```python
from build123d import *

# Parameters (mm, degrees)
BOSS_EXTRUDE1_DEPTH       = 53.2
SKETCH2_W                 = 95
SKETCH2_H                 = 20
BOSS_EXTRUDE2_DEPTH       = 3.5
CHAMFER1_SIZE             = 50
CHAMFER1_SIZE2            = 10
SKETCH3_W                 = 89
SKETCH3_H                 = 19
BOSS_EXTRUDE3_DEPTH       = 3.5
BOSS_EXTRUDE4_START       = -3.5
BOSS_EXTRUDE4_DEPTH       = 6
FILLET1_R                 = 5
F_2_5MM_DOWEL_HOLE1_D     = 3.2
F_2_5MM_DOWEL_HOLE1_DEPTH = 6.5
F_2_5MM_DOWEL_HOLE1_TIP   = 0.96137699


with BuildPart() as part:
    # Sketch1 → Boss-Extrude1 (new body)
    with BuildSketch(Plane.XY):
        Polygon((-60.5, 15), (-60.5, 20), (-57.5, 20), (-57.5, 0), (-152.5, 0), (-152.5, 20), (-149.5, 20), (-149.5, 15), align=None)
    extrude(amount=BOSS_EXTRUDE1_DEPTH)

    # Sketch2 → Boss-Extrude2 (add)
    with BuildSketch(Plane.XY.offset(53.2)):
        with Locations((-105, 10)):
            Rectangle(SKETCH2_W, SKETCH2_H)
    extrude(amount=BOSS_EXTRUDE2_DEPTH)

    # Chamfer1
    chamfer1_edges = [part.edges().sort_by_distance(p)[0] for p in [
        (-105, 0, 56.7),
    ]]
    chamfer1_side = [part.faces().sort_by_distance(p)[0] for p in [
        (-105, 0, 28.35),
    ]]
    chamfer(chamfer1_edges, length=CHAMFER1_SIZE, length2=CHAMFER1_SIZE2, reference=chamfer1_side[0])

    # Sketch3 → Boss-Extrude3 (add)
    with BuildSketch(Plane.XY.offset(56.7)):
        with Locations((-105, 29.5)):
            Rectangle(SKETCH3_W, SKETCH3_H)
        Polygon((-152.5, 42.463842296), (-152.5, 20), (-149.5, 20), (-149.5, 39), (-60.5, 39), (-60.5, 20), (-57.5, 20), (-57.5, 42.463842296), align=None)
    extrude(amount=-BOSS_EXTRUDE3_DEPTH)

    # Sketch3<3> → Boss-Extrude4 (add)
    with BuildSketch(Plane.XY.offset(56.7).offset(BOSS_EXTRUDE4_START)):
        Polygon((-152.5, 42.463842296), (-152.5, 20), (-149.5, 20), (-149.5, 39), (-60.5, 39), (-60.5, 20), (-57.5, 20), (-57.5, 42.463842296), align=None)
    extrude(amount=-BOSS_EXTRUDE4_DEPTH)

    # Fillet1
    fillet1_edges = [part.edges().sort_by_distance(p)[0] for p in [
        (-151, 20, 47.2),
        (-59, 20, 47.2),
    ]]
    fillet(fillet1_edges, radius=FILLET1_R)

    # Ø2.5mm Dowel Hole1
    with Locations(Plane(origin=(0, 0, 0), x_dir=(-1, 0, 0), z_dir=(0, 0, -1))):
        with Locations((70, 5.6), (140, 5.6)):
            Hole(F_2_5MM_DOWEL_HOLE1_D / 2, depth=F_2_5MM_DOWEL_HOLE1_DEPTH)
            with Locations((0, 0, -(F_2_5MM_DOWEL_HOLE1_DEPTH + F_2_5MM_DOWEL_HOLE1_TIP / 2))):  # 118° drill point
                Cone(0, F_2_5MM_DOWEL_HOLE1_D / 2, F_2_5MM_DOWEL_HOLE1_TIP, mode=Mode.SUBTRACT)


solid = part.part
```
Check sheet for the modelled part. Datum: model origin and axes. Units: mm. A direction names the side the tool comes from. Round coordinates to 2 decimals unless told otherwise and drop trailing zeros. Write each loop counter-clockwise with the first axis right and the second up, starting at its lowest first coordinate (ties: lowest second). Pieces come first, ordered by that corner, then holes. Notation, with made-up numbers: (20.25, 87.25) -> (39.25, 87.25) arc R20 cw to (39.25, 91.25) -> close; hole circle Ø10 at (10, 50). An arc over 180 degrees is marked (long way). One line per question, with ' | ' between items. Start each with the question number.
1. Sectioned sample at C-C, the plane y = 21. Record the cut outline in (x, z), then the cut area to 4 significant figures.
2. Set-up check for faces 1 (the face through (-106, 0, 3)), 2 (the face through (-151, 20, 21)), 3 (the face through (-106, 39, 50)): record each of +Z, -Z, +X, -X, +Y, -Y from which the full face is reachable in a straight line by a thin tool's end or side.
3. Sectioned sample at B-B, the plane x = -118. Record the cut outline in (y, z), then the cut area to 3 significant figures.
4. Sectioned sample at D-D, the plane z = 39. Record the cut outline in (x, y).
5. Sectioned sample at A-A, the plane z = 50. Record the cut outline in (x, y), then the cut area to 3 significant figures.
6. Release check for a two-part mould opening along X. For faces 4 (the face through (-58.98, 21.43, 45.7)), 5 (the face through (-152.5, 17, 35)), 6 (the face through (-106, 27, 53.2)) record: +X half, -X half, draft (parallel to the pull), parting line (faces both ways), or undercut.
7. Depth check by flat-ended pin: pin 1 (5 mm diameter, centred on x = -86.5, z = 50, fed in from -Y); pin 2 (19 mm diameter, centred on x = -100.5, y = 37.5, fed in from -Z); pin 3 (4 mm diameter, centred on x = -97, z = 25.5, fed in from +Y). Enter the tip coordinate at first touch or a pass-through.
8. Scan lines: line 1 along X through (y, z) = (5.6, 2.75); line 2 along Y through (x, z) = (-70, 3); line 3 along X through (y, z) = (37, 49). Record each from-to range of solid material in increasing order. Write a range as from..to.
Taken from the geometry:
1) outline: (-152.5, 45.2) -> (-149.5, 45.2) -> (-149.5, 53.2) -> (-60.5, 53.2) -> (-60.5, 45.2) -> (-57.5, 45.2) -> (-57.5, 56.7) -> (-152.5, 56.7) -> close | area: 380.5 mm^2
2) face 1: +Z, -Z, +X, -X, -Y | face 2: -Z, +X, -X, +Y | face 3: -Z
3) outline: (0, 0) -> (15, 0) -> (15, 53.2) -> (39, 53.2) -> (39, 47.2) -> (42.46, 47.2) -> (42.46, 56.7) -> (10, 56.7) -> (0, 6.7) -> close | area: 717 mm^2
4) outline: (-152.5, 6.46) -> (-57.5, 6.46) -> (-57.5, 20) -> (-60.5, 20) -> (-60.5, 15) -> (-149.5, 15) -> (-149.5, 20) -> (-152.5, 20) -> close
5) outline: (-152.5, 8.66) -> (-57.5, 8.66) -> (-57.5, 42.46) -> (-152.5, 42.46) -> close; hole (-149.5, 15) -> (-60.5, 15) -> (-60.5, 39) -> (-149.5, 39) -> close | area: 1,080 mm^2
6) face 4: draft | face 5: -X half | face 6: undercut
7) pin 1: stops at y = 8.16 | pin 2: stops at z = 47.2 | pin 3: stops at y = 15
8) line 1: x = -152.5..-141.6, -138.4..-71.6, -68.4..-57.5 | line 2: y = 0..4, 7.2..15 | line 3: x = -152.5..-149.5, -60.5..-57.5
